Part model, mm, in its own coordinate system. A direction names the side the tool comes from. Coordinates: 2 decimals unless noted, no trailing zeros. Loops run counter-clockwise (first coordinate to the right, second up) from the corner with the lowest first, then second, coordinate; pieces in that order, holes last. Notation, with made-up numbers: M 73.5,48 L 89.5,48 A15 ccw 89.5,73 Z; hole C 40,50 d8. An arc over 180 degrees is marked long. Use a Markdown table: item, result. Add a question column.
1) Band-saw the part on A-A (y = -2.25). List the corners of the cut face in (x, z).
2) Band-saw the part on B-B (x = -23.5). List the corners of the cut face in (y, z).
3) Wall check: probe 1 along Z at (x, y) = (15.5, -3); probe 2 along Y at (x, z) = (-11, -8). Give the ranges that are in metal, low to high. Write a range as from..to.
4) Pin check, flat tip, straight feed: pin 1 Ø5 at (x, z) = (14.5, 20.5) entering from -Y. Stop position of the tip, or through.
5) Band-saw the part on C-C (z = -7.5). List the corners of the cut face in (x, y), plus the area to 3 significant figures.
6) Pull direction X, two halves, no side cores. Call faces 1 (the flat face through (0, 0, -40.5)), 2 (the cylindrical face through (-39.07, -0.06, -39)), 3 (the flat face through (-36.5, -2, 0)), 4 (the cylindrical face through (-35.297, -1.972, -35.359)): released by +X, released by -X, zero draft, split by the parting line, or undercut.
7) Tool access for faces 5 (the cylindrical face through (27.6, -2, -31.5)), 6 (the cylindrical face through (-39.07, 0.06, 39)): list every direction of +Z, -Z, +X, -X, +Y, -Y with a clear straight run to the whole face (end or side of a thin tool).
from build123d import *

# Parameters (mm, degrees)
SKETCH2_W           = 81
SKETCH2_H           = 81
BOSS_EXTRUDE1_DEPTH = 4
CUT_EXTRUDE1_DEPTH  = 4
FILLET1_R           = 5


with BuildPart() as part:
    # Sketch2 → Boss-Extrude1 (new body, symmetric)
    with BuildSketch(Plane(origin=(0, 0, 0), x_dir=(1, 0, 0), z_dir=(0, 1, 0))):
        Rectangle(SKETCH2_W, SKETCH2_H)
    extrude(amount=BOSS_EXTRUDE1_DEPTH, both=True)

    # Sketch1 → Cut-Extrude1 (cut)
    with BuildSketch(Plane(origin=(0, 0, 0), x_dir=(1, 0, 0), z_dir=(0, 1, 0))):
        with BuildLine():
            Line((22.5, 36.5), (-32.5, 36.5))
            ThreePointArc((-32.5, 36.5), (-35.328427125, 35.328427125), (-36.5, 32.5))
            Line((-36.5, 32.5), (-36.5, -32.5))
            ThreePointArc((-36.5, -32.5), (-35.328427125, -35.328427125), (-32.5, -36.5))
            Line((-32.5, -36.5), (32.5, -36.5))
            ThreePointArc((32.5, -36.5), (35.328427125, -35.328427125), (36.5, -32.5))
            Line((36.5, -32.5), (36.5, 32.5))
            ThreePointArc((36.5, 32.5), (35.328427125, 35.328427125), (32.5, 36.5))
            ThreePointArc((32.5, 36.5), (27.5, 31.5), (22.5, 36.5))
        make_face()
    extrude(amount=-CUT_EXTRUDE1_DEPTH, mode=Mode.SUBTRACT)

    # Fillet1
    fillet1_edges = [part.edges().sort_by_distance(p)[0] for p in [
        (-40.5, 0, 40.5),
        (-40.5, 0, -40.5),
        (40.5, 0, -40.5),
        (40.5, 0, 40.5),
    ]]
    fillet(fillet1_edges, radius=FILLET1_R)


solid = part.part
Entries:
| question | item | result |
|---|---|---|
| 1 | outline | M -40.5,-35.5 A5 ccw -35.5,-40.5 L 35.5,-40.5 A5 ccw 40.5,-35.5 L 40.5,35.5 A5 ccw 35.5,40.5 L -35.5,40.5 A5 ccw -40.5,35.5 Z; hole M -36.5,-32.5 A4 ccw -32.5,-36.5 L 22.5,-36.5 A5 cw 32.5,-36.5 A4 ccw 36.5,-32.5 L 36.5,32.5 A4 ccw 32.5,36.5 L -32.5,36.5 A4 ccw -36.5,32.5 Z |
| 2 | outline | M -4,-40.5 L 4,-40.5 L 4,40.5 L -4,40.5 L -4,36.5 L 0,36.5 L 0,-36.5 L -4,-36.5 Z |
| 3 | probe 1 | -40.5..-36.5, 36.5..40.5 |
| 3 | probe 2 | 0..4 |
| 4 | pin 1 | y = 0 |
| 5 | outline | M -40.5,-4 L -36.5,-4 L -36.5,0 L 36.5,0 L 36.5,-4 L 40.5,-4 L 40.5,4 L -40.5,4 Z |
| 5 | area | 356 mm2 |
| 6 | face 1 | zero draft |
| 6 | face 2 | released by -X |
| 6 | face 3 | undercut |
| 6 | face 4 | undercut |
| 7 | face 5 | -Y |
| 7 | face 6 | +Z, -X, +Y, -Y |
